Build history of the part. All positions in model axes, mm. A direction names the side the tool comes from. Coordinates: 2 decimals unless noted, no trailing zeros. Order: outer loops, then holes, each group sorted by start corner. A loop starts at its lowest first (then second) coordinate and runs counter-clockwise, first axis right, second up. Notation, with made-up numbers: (-39, -11) - (-31, -11) arc R10 ccw to (-31, -1) - close; hole circle Ø11 at (39.5, 27.5). An arc over 180 degrees is marked (long way). Write each question's results on one line, items separated by ' | '.
Autodesk Inventor part; units mm, degrees
ref_plane "YZ Plane" through (0, 0, 0) normal (1, 0, 0) x (0, 1, 0)
ref_plane "XZ Plane" through (0, 0, 0) normal (0, 1, 0) x (-1, 0, 0)
ref_plane "XY Plane" through (0, 0, 0) normal (0, 0, 1) x (1, 0, 0)
sketch "Sketch2" plane through (0, 0, 0) normal (0, 1, 0) x (-1, 0, 0)
  circle A0 centre (0, 0) radius 15.25
  circle A1 centre (0, 0) radius 25 construction
  circle A2 centre (0, -105) radius 68.1
  line L0 (-85.4561, 0) -> (89.9732, 0) construction
  line L1 (0, 101.2907) -> (0, -205.3562) construction
  circle A3 centre (0, -105) radius 72
  line L2 (53.1573, -36.9) -> (-40.009, -36.9) construction
  line L3 (26.7586, 36.9) -> (26.7586, -36.9)
  line L4 (-26.7586, 36.9) -> (-26.7586, -36.9)
  line L5 (26.7586, -36.9) -> (-26.7586, -36.9)
  line L6 (34.2741, -33.2) -> (-37.5386, -33.2) construction
  line L7 (0, 0) -> (20, 0)
  line L8 (0, 0) -> (-10, 17.3205)
  line L9 (0, 0) -> (-10, -17.3205)
  line L10 (0, 17.3205) -> (-18.0278, 17.3205) construction
  line L11 (0, -17.3205) -> (-18.0278, -17.3205) construction
  circle A4 centre (-10, 17.3205) radius 2.1
  circle A5 centre (20, 0) radius 2.1
  circle A6 centre (-10, -17.3205) radius 2.1
  line L12 (26.7586, 36.9) -> (-26.7586, 36.9)
  dimension "d22" = 30.5
  dimension "d23" = 50
  dimension "d24" = 136.2
  dimension "d25" = 105
  dimension "d26" = 144
  dimension "d40" = 120
  dimension "d41" = 120
  dimension "d42" = 20
  dimension "d43" = 4.2
sketch "Sketch4" plane through (0, 0, 0) normal (0, 1, 0) x (-1, 0, 0)
  line L0 (0, 0) -> (29, 0)
  line L1 (29, 0) -> (29, 3.2)
  line L2 (29, 3.2) -> (26, 3.2)
  line L3 (26, 3.2) -> (26, 6.2)
  line L4 (26, 6.2) -> (34.5, 6.2)
  line L5 (34.5, 6.2) -> (34.5, -2.8)
  line L6 (34.5, -2.8) -> (32, -2.8)
  line L7 (32, -2.8) -> (32, -6)
  line L8 (32, -6) -> (0, -6)
  line L9 (0, -6) -> (0, 0)
  line L10 (0, 0) -> (-29, 0)
  line L11 (-29, 0) -> (-29, 3.2)
  line L12 (-29, 3.2) -> (-26, 3.2)
  line L13 (-26, 3.2) -> (-26, 6.2)
  line L14 (-26, 6.2) -> (-34.5, 6.2)
  line L15 (-34.5, 6.2) -> (-34.5, -2.8)
  line L16 (-34.5, -2.8) -> (-32, -2.8)
  line L17 (-32, -2.8) -> (-32, -6)
  line L18 (-32, -6) -> (0, -6)
  dimension "d44" = 3.2
  dimension "d45" = 3.2
  dimension "d46" = 6
  dimension "d47" = 3
  dimension "d48" = 3
  dimension "d49" = 5.5
  dimension "d50" = 3
  dimension "d51" = 26
extrude "Extrusion1" add sketch "Sketch4" along normal blind 80
sketch "Sketch6" plane through (-29, 0, 0) normal (0, 0, 1) x (1, 0, 0)
  line L0 (0, 80) -> (58, 80)
  line L1 (0, 0) -> (0, 80)
  line L2 (0, 0) -> (58, 0)
  line L3 (0, 0) -> (58, 0)
  line L4 (58, 0) -> (58, 80)
  line L5 (58, 0) -> (58, 80)
  circle A0 centre (29, 40) radius 25 construction
  line L6 (36.5497, 40) -> (21.3269, 40) construction
  line L7 (29, 31.55) -> (29, 50.9237) construction
  line L8 (29, 40) -> (39, 57.3205) construction
  line L9 (29, 40) -> (9, 40) construction
  line L10 (29, 40) -> (39, 22.6795) construction
  circle A1 centre (29, 40) radius 15.25
  point P0 (29, 0)
  dimension "d54" = 50
  dimension "d56" = 120
  dimension "d57" = 120
  dimension "d58" = 20
  dimension "d59" = 30.5
extrude "Extrusion2" cut sketch "Sketch6" against normal up to surface (6 mm away) contours A1
hole "Hole1" at (10, 22.6795, 0) at (-20, 40, 0) at (10, 57.3205, 0) direction (0, 0, -1) diameter 4.2 end through all countersink diameter 8 countersink angle 90
properties part number "Cycloid_2_base_v2"
1. Band-saw the part on A-A on y = 40. Give the cut face in (x, z).
Solved:
outline: (-34.5, -2.8) - (-32, -2.8) - (-32, -6) - (-22.1, -6) - (-22.1, -1.9) - (-24, 0) - (-29, 0) - (-29, 3.2) - (-26, 3.2) - (-26, 6.2) - (-34.5, 6.2) - close; (-17.9, -6) - (-15.25, -6) - (-15.25, 0) - (-16, 0) - (-17.9, -1.9) - close; (15.25, -6) - (32, -6) - (32, -2.8) - (34.5, -2.8) - (34.5, 6.2) - (26, 6.2) - (26, 3.2) - (29, 3.2) - (29, 0) - (15.25, 0) - close
2. Band-saw the part on D-D on y = 50. Give the cut face in (x, z).
Solved:
outline: (-34.5, -2.8) - (-32, -2.8) - (-32, -6) - (-11.51, -6) - (-11.51, 0) - (-29, 0) - (-29, 3.2) - (-26, 3.2) - (-26, 6.2) - (-34.5, 6.2) - close; (11.51, -6) - (32, -6) - (32, -2.8) - (34.5, -2.8) - (34.5, 6.2) - (26, 6.2) - (26, 3.2) - (29, 3.2) - (29, 0) - (11.51, 0) - close
3. Tool access for faces 1 (the face through (26, 39, 5)), 2 (the face through (-33, 39, -2.8)), 3 (the face through (-12.5, 30.6, 0)): list every direction of +Z, -Z, +X, -X, +Y, -Y with a clear straight run to the whole face (end or side of a thin tool).
Solved:
face 1: +Z, +Y, -Y | face 2: -Z, -X, +Y, -Y | face 3: +Y, -Y
4. Band-saw the part on C-C on x = 0. Give the cut face in (y, z), then the cut area to 3 significant figures.
Solved:
outline: (0, -6) - (24.75, -6) - (24.75, 0) - (0, 0) - close; (55.25, -6) - (80, -6) - (80, 0) - (55.25, 0) - close | area: 297 mm2
5. Probe line 1 (X direction, y = 14.5, z = 1.5); line 2 (Y direction, x = 10, z = -4.25); line 3 (Z direction, x = 28, y = 4.5). List the from-to ranges inside material, lowest first.
Solved:
line 1: x = -34.5 to -29, 29 to 34.5 | line 2: y = 0 to 20.58, 24.78 to 28.49, 51.51 to 55.22, 59.42 to 80 | line 3: z = -6 to 0, 3.2 to 6.2
6. Drop flat-ended pins along their axis: pin 1 Ø2.5 at (y, z) = (41, -5) entering from -X; pin 2 Ø5 at (x, z) = (-19.5, 2) entering from +Y; pin 3 Ø5 at (x, y) = (17.5, 50) entering from +Z; pin 4 Ø2 at (x, y) = (33.5, 29.5) entering from -Z. Give the stop position or say it passes through.
Solved:
pin 1: stops at x = -32 | pin 2: stops at y = 80 | pin 3: stops at z = 0 | pin 4: stops at z = -2.8
7. Two-plate mould, pull along X, no slides. Class faces 4 (the face through (30, 39, 6.2)), 5 (the face through (32, 39, -4)), 6 (the face through (-26, 39, 5)): +X half, -X half, draft (parallel to the pull), parting line (faces both ways), or undercut.
Solved:
face 4: draft | face 5: +X half | face 6: undercut
8. Band-saw the part on B-B on z = 1. Give the cut face in (x, y).
Solved:
outline: (-34.5, 0) - (-29, 0) - (-29, 80) - (-34.5, 80) - close; (29, 0) - (34.5, 0) - (34.5, 80) - (29, 80) - close
